The model under review builds one solid part; all positions refer to its coordinate system, in mm. A direction names the side the tool comes from. Give positions to 0.01 mm unless a question says otherwise; leave off trailing zeros. Loops run counter-clockwise (first coordinate to the right, second up) from the corner with the lowest first, then second, coordinate; pieces in that order, holes last. Notation, with made-up numbers: M 59.25,62.5 L 69.25,62.5 A6 ccw 69.25,68.5 Z; hole C -16,49 d1. An arc over 180 degrees is marked long. Return JSON: item names as keys, results as strings.
```python
from build123d import *

# Parameters (mm, degrees)
F0_R     = 10
F0_R_2   = 4.3
F1_DEPTH = 13
F2_R     = 4.3
F3_DEPTH = 3
F6_DEPTH = 25.4
F7_R     = 1.5
F8_DEPTH = 25.4


with BuildPart() as f1:
    # F0 (on Top) → F1 (new body)
    with BuildSketch(Plane.XY):
        Circle(F0_R)
        Circle(F0_R_2, mode=Mode.SUBTRACT)
    extrude(amount=F1_DEPTH)

    # F2 (on Top) → F3 (join)
    with BuildSketch(Plane.XY):
        Circle(F2_R)
    extrude(amount=F3_DEPTH)

    # F5 (on offset) → F6 (cut)
    with BuildSketch(Plane.XY.offset(13)):
        with BuildLine():
            ThreePointArc((0, -5.5), (-1.5, -7), (0, -8.5))
            Line((0, -8.5), (0, -5.5))
        make_face()
        with BuildLine():
            ThreePointArc((0, 8.5), (-1.5, 7), (0, 5.5))
            Line((0, 5.5), (0, 8.5))
        make_face()
        with BuildLine():
            Line((0, 8.5), (0, 5.5))
            ThreePointArc((0, 5.5), (1.06066, 5.93934), (1.5, 7))
            ThreePointArc((1.5, 7), (1.06066, 8.06066), (0, 8.5))
        make_face()
        with BuildLine():
            Line((0, -5.5), (0, -8.5))
            ThreePointArc((0, -8.5), (1.06066, -8.06066), (1.5, -7))
            ThreePointArc((1.5, -7), (1.06066, -5.93934), (0, -5.5))
        make_face()
    extrude(amount=-F6_DEPTH, mode=Mode.SUBTRACT)

    # F7 (on Right) → F8 (cut)
    with BuildSketch(Plane.YZ):
        with Locations((0, 5)):
            Circle(F7_R)
    extrude(amount=-F8_DEPTH, mode=Mode.SUBTRACT)


solid = f1.part
```
1) Consider section A-A on y = 0. Write out the cut boundary in (x, z), then the cut area to 3 significant figures.
From the geometry:
{"outline": "M -10,0 L 10,0 L 10,13 L 4.3,13 L 4.3,3 L -4.3,3 L -4.3,3.5 L -10,3.5 Z; M -10,6.5 L -4.3,6.5 L -4.3,13 L -10,13 Z", "area": "157 mm²"}
2) The part is to be moulded in two halves that separate along Z. For faces 1 (the face through (0, 0, 3)), 2 (the face through (-6.97, -1.5, 5.07)), 3 (the face through (0, 0, 0)), say which applies: released by +Z, released by -Z, zero draft, split by the parting line, or undercut.
From the geometry:
{"face 1": "released by +Z", "face 2": "undercut", "face 3": "released by -Z"}
3) Tool access review of faces 4 (the face through (4.1, 1.3, 7.9)), 5 (the face through (9.54, 3, 6.41)): name each direction out of +Z, -Z, +X, -X, +Y, -Y from which nothing blocks a thin tool from reaching the whole face with its end or side.
From the geometry:
{"face 4": "+Z", "face 5": "+Z, -Z"}
4) Wall thickness on L1, parallel to X at y = 0, z = 9; L2, parallel to Z at x = 3.75, y = -1.75; L3, parallel to X at y = 0.75, z = 6.5: over which ranges is each line inside the solid? List them lowest first. Write a range as from..to.
From the geometry:
{"L1": "-10..-4.3, 4.3..10", "L2": "0..3", "L3": "-9.97..-4.23, 4.23..9.97"}
5) Consider section C-C on x = -8. Write out the cut boundary in (y, z).
From the geometry:
{"outline": "M -6,0 L 6,0 L 6,13 L -6,13 Z; hole C 0,5 d3"}
6) Consider section B-B on z = 9. Write out the cut boundary in (x, y).
From the geometry:
{"outline": "C 0,0 d20; hole C 0,0 d8.6; hole M 0,-5.5 A1.5 ccw long 1.5,-7 A1.5 ccw Z; hole M 0,8.5 A1.5 ccw long 1.5,7 A1.5 ccw Z"}
7) Consider section D-D on x = -0.25. Write out the cut boundary in (y, z), then the cut area to 3 significant figures.
From the geometry:
{"outline": "M -10,0 L -8.48,0 L -8.48,13 L -10,13 Z; M -5.52,0 L 5.52,0 L 5.52,13 L 4.29,13 L 4.29,3 L -4.29,3 L -4.29,13 L -5.52,13 Z; M 8.48,0 L 10,0 L 10,13 L 8.48,13 Z", "area": "97.2 mm²"}
8) Insertion check: pin 1 (4 mm diameter, centred on y = -3.5, z = 4.5, fed in from -X); pin 2 (4 mm diameter, centred on x = -6.5, z = 6.5, fed in from +Y); pin 3 (2.5 mm diameter, centred on x = 1, y = -0.5, fed in from +Z). Each pin has a flat end and moves straight along its axis. Give the tip position at first contact, or say it passes through.
From the geometry:
{"pin 1": "x = -9.89", "pin 2": "y = 8.93", "pin 3": "z = 3"}
